Read the model definition and answer for the solid it produces. Units are mm, in the model's axes. Give positions to 0.01 mm unless a question says otherwise; leave off trailing zeros. Order: outer loops, then holes, each group sorted by start corner. A loop starts at its lowest first (then second) coordinate and runs counter-clockwise, first axis right, second up. Notation, with made-up numbers: (56.25, 61.25) - (103.25, 61.25) arc R36 ccw to (103.25, 96.25) - close; hole circle Ø7 at (16, -29). An arc over 180 degrees is marked (long way). Write each question's results on one line, items separated by ' | '. Start each with the question number.
Q1. Find section B-B on z = 3.75. Count the separate pieces of the cut face and the enclosed holes in it, and give its area (3 significant figures).
Q2. Find section A-A on x = -168.5. Give the vertices of the cut face in (y, z).
Q3. Find the intervals of material crossed by line 1 along Y through (x, z) = (26.5, 3.9), in increasing order. Write a range as from..to.
from build123d import *

# Parameters (mm, degrees)
SKETCH1_W           = 600
SKETCH1_H           = 200
EXTRUDE1_DEPTH      = 5
CUT_EXTRUDE1_REACH  = 362.59
SKETCH2_W           = 350
SKETCH2_H           = 20
CUT_EXTRUDE2_REACH  = 362.59
SKETCH4_W           = 5
SKETCH4_H           = 5
LPATTERN4_COUNT     = 5
LPATTERN4_PITCH     = 50
LPATTERN4_COL_COUNT = 5
LPATTERN4_COL_PITCH = 50


with BuildPart() as part:
    # Sketch1 → Extrude1 (new body)
    with BuildSketch(Plane.XY):
        with Locations((0, 100)):
            Rectangle(SKETCH1_W, SKETCH1_H)
    extrude(amount=EXTRUDE1_DEPTH)

    # Sketch2 → Cut-Extrude1 (cut, up to next)
    with BuildSketch(Plane.XY.offset(5), mode=Mode.PRIVATE) as cut_extrude1_sk1:
        with Locations((0, 150)):
            Rectangle(SKETCH2_W, SKETCH2_H)
    cut_extrude1_tool1 = extrude(cut_extrude1_sk1.sketch, amount=-CUT_EXTRUDE1_REACH, mode=Mode.PRIVATE) & part.part
    add(cut_extrude1_tool1.solids().sort_by_distance((0, 150, 5))[0], mode=Mode.SUBTRACT)

    # Sketch4 → Cut-Extrude2 (cut, up to next)
    with BuildSketch(Plane.XY.offset(5), mode=Mode.PRIVATE) as cut_extrude2_sk1:
        with Locations((0, 67.5)):
            Rectangle(SKETCH4_W, SKETCH4_H)
    cut_extrude2_tool1 = extrude(cut_extrude2_sk1.sketch, amount=-CUT_EXTRUDE2_REACH, mode=Mode.PRIVATE) & part.part
    # Sketch4 → Cut-Extrude2 (cut, up to next)
    with BuildSketch(Plane.XY.offset(5), mode=Mode.PRIVATE) as cut_extrude2_sk2:
        with Locations((0, 92.5)):
            Rectangle(SKETCH4_W, SKETCH4_H)
    cut_extrude2_tool2 = extrude(cut_extrude2_sk2.sketch, amount=-CUT_EXTRUDE2_REACH, mode=Mode.PRIVATE) & part.part
    cut_extrude2_1 = cut_extrude2_tool1.solids().sort_by_distance((0, 67.5, 5))[0]
    add(cut_extrude2_1, mode=Mode.SUBTRACT)
    cut_extrude2_2 = cut_extrude2_tool2.solids().sort_by_distance((0, 92.5, 5))[0]
    add(cut_extrude2_2, mode=Mode.SUBTRACT)
    cut_extrude2 = cut_extrude2_1 + cut_extrude2_2  # Cut-Extrude2 as one shape, for the pattern or mirror that repeats it

    # LPattern4: Cut-Extrude2 ×5
    with Locations(*[(-i * LPATTERN4_PITCH, 0, 0) for i in range(1, LPATTERN4_COUNT)]):
        add(cut_extrude2, mode=Mode.SUBTRACT)

    # LPattern4 col: Cut-Extrude2 ×5
    with Locations(*[(i * LPATTERN4_COL_PITCH, 0, 0) for i in range(1, LPATTERN4_COL_COUNT)]):
        add(cut_extrude2, mode=Mode.SUBTRACT)


solid = part.part
Working result:
1) separate pieces: 1 | enclosed holes: 19 | area: 113,000 mm²
2) outline: (0, 0) - (140, 0) - (140, 5) - (0, 5) - close; (160, 0) - (200, 0) - (200, 5) - (160, 5) - close
3) line 1: 0..140, 160..200
